Source: CAD feature listing. Evaluate the final solid. Frame: model axes, mm. Round coordinates to 2 decimals unless told otherwise and drop trailing zeros. Order: outer loops, then holes, each group sorted by start corner. A loop starts at its lowest first (then second) coordinate and runs counter-clockwise, first axis right, second up. Notation, with made-up numbers: (-27.75, -10.75) - (11.25, -10.75) arc R27 ccw to (11.25, 26.25) - close; hole circle Ø10 at (16, 73). An arc over 180 degrees is marked (long way). Return JSON: item names as keys, results as strings. Group by question number.
1) Section A-A, the plane x = -17. Return loops of the section in (y, z), plus the area to 3 significant figures.
2) Contact query for flat-ended pins moving along their axis: P1, Ø1.9, axis at y = 10, z = 1.5, coming from the +X side; P2, Ø1.9, axis at x = -18, z = 2, coming from the +Y side; P3, Ø1.9, axis at x = -51, z = 4, coming from the -Y side. Output: stop coordinate, or through.
3) Ray query, line 1 (X direction, y = 30.5, z = 0.5); line 2 (Y direction, x = -3.5, z = 3.5); line 3 (Y direction, x = -29.5, z = 1.5). Return the intervals inside material, ascending. Write a range as from..to.
4) Section B-B, the plane y = -8. Return loops of the section in (x, z), plus the area to 3 significant figures.
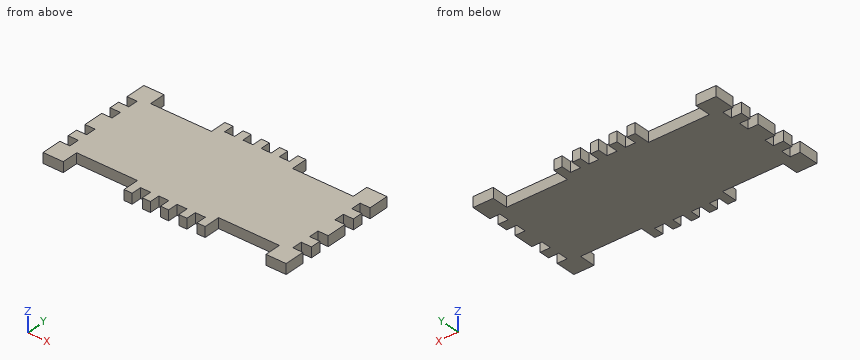
```python
from build123d import *

# Parameters (mm, degrees)
F1_DEPTH = 6.35


with BuildPart() as f1:
    # F0 (on Top) → F1 (new body)
    with BuildSketch(Plane.XY):
        Polygon((-76.2, 0), (0, 0), (0, 38.1), (-2.54, 38.1), (-2.54, 31.75), (-8.89, 31.75), (-8.89, 38.1), (-13.97, 38.1), (-13.97, 31.75), (-20.32, 31.75), (-20.32, 38.1), (-25.4, 38.1), (-25.4, 27.94), (-63.5, 27.94), (-63.5, 38.1), (-76.2, 38.1), (-76.2, 25.4), (-69.85, 25.4), (-69.85, 19.05), (-76.2, 19.05), (-76.2, 12.7), (-69.85, 12.7), (-69.85, 6.35), (-76.2, 6.35), align=None)
        Polygon((0, -38.1), (0, 0), (-76.2, 0), (-76.2, -6.35), (-69.85, -6.35), (-69.85, -12.7), (-76.2, -12.7), (-76.2, -19.05), (-69.85, -19.05), (-69.85, -25.4), (-76.2, -25.4), (-76.2, -38.1), (-63.5, -38.1), (-63.5, -27.94), (-25.4, -27.94), (-25.4, -38.1), (-20.32, -38.1), (-20.32, -31.75), (-13.97, -31.75), (-13.97, -38.1), (-8.89, -38.1), (-8.89, -31.75), (-2.54, -31.75), (-2.54, -38.1), align=None)
        Polygon((63.5, -38.1), (76.2, -38.1), (76.2, -25.4), (69.85, -25.4), (69.85, -19.05), (76.2, -19.05), (76.2, -12.7), (69.85, -12.7), (69.85, -6.35), (76.2, -6.35), (76.2, 0), (0, 0), (0, -38.1), (2.54, -38.1), (2.54, -31.75), (8.89, -31.75), (8.89, -38.1), (13.97, -38.1), (13.97, -31.75), (20.32, -31.75), (20.32, -38.1), (25.4, -38.1), (25.4, -27.94), (63.5, -27.94), align=None)
        Polygon((0, 0), (76.2, 0), (76.2, 6.35), (69.85, 6.35), (69.85, 12.7), (76.2, 12.7), (76.2, 19.05), (69.85, 19.05), (69.85, 25.4), (76.2, 25.4), (76.2, 38.1), (63.5, 38.1), (63.5, 27.94), (25.4, 27.94), (25.4, 38.1), (20.32, 38.1), (20.32, 31.75), (13.97, 31.75), (13.97, 38.1), (8.89, 38.1), (8.89, 31.75), (2.54, 31.75), (2.54, 38.1), (0, 38.1), align=None)
    extrude(amount=F1_DEPTH)


solid = f1.part
```
Geometry check:
{
 "1": {"outline": "(-31.75, 0) - (31.75, 0) - (31.75, 6.35) - (-31.75, 6.35) - close", "area": "403 mm2"},
 "2": {"P1": "x = 69.85", "P2": "y = 31.75", "P3": "y = -27.94"},
 "3": {"line 1": "-76.2..-63.5, -25.4..25.4, 63.5..76.2", "line 2": "-31.75..31.75", "line 3": "-27.94..27.94"},
 "4": {"outline": "(-69.85, 0) - (69.85, 0) - (69.85, 6.35) - (-69.85, 6.35) - close", "area": "887 mm2"}
}
